from build123d import *

# Parameters (mm, degrees)
SKETCH1_W           = 29.9
SKETCH1_H           = 12.55
SKETCH1_R           = 1.5
BOSS_EXTRUDE1_DEPTH = 3.175
SKETCH2_W           = 29.9
SKETCH2_H           = 12.55
BOSS_EXTRUDE2_DEPTH = 3.175
BOSS_EXTRUDE3_DEPTH = 55.88
BOSS_EXTRUDE4_DEPTH = 3.175
SKETCH6_W           = 25.9
SKETCH6_H           = 8.55
CUT_EXTRUDE1_DEPTH  = 57.23
SKETCH7_W           = 23.9
SKETCH7_H           = 49.88
CUT_EXTRUDE2_DEPTH  = 23.211


with BuildPart() as part:
    # Sketch1 → Boss-Extrude1 (new body)
    # profile 1 of 3: a face of its own
    with BuildSketch(Plane.XY):
        with Locations((14.95, 6.275)):
            Rectangle(SKETCH1_W, SKETCH1_H)
    # profile 2 of 3: a face of its own
    with BuildSketch(Plane.XY):
        with BuildLine():
            Line((-5, 6.275), (0, 6.275))
            Line((0, 6.275), (0, 12.55))
            Line((0, 12.55), (-5, 12.55))
            ThreePointArc((-5, 12.55), (-8.1375, 9.4125), (-5, 6.275))
        make_face()
        with Locations((-5, 9.4125)):
            Circle(SKETCH1_R, mode=Mode.SUBTRACT)
    # profile 3 of 3: a face of its own
    with BuildSketch(Plane.XY):
        with BuildLine():
            Line((29.9, 12.55), (29.9, 6.275))
            Line((29.9, 6.275), (34.9, 6.275))
            ThreePointArc((34.9, 6.275), (38.0375, 9.4125), (34.9, 12.55))
            Line((34.9, 12.55), (29.9, 12.55))
        make_face()
        with Locations((34.9, 9.4125)):
            Circle(SKETCH1_R, mode=Mode.SUBTRACT)
    extrude(amount=BOSS_EXTRUDE1_DEPTH)

    # Sketch2 → Boss-Extrude2 (add)
    with BuildSketch(Plane.XY.offset(3.175)):
        with Locations((14.95, 6.275)):
            Rectangle(SKETCH2_W, SKETCH2_H)
    extrude(amount=BOSS_EXTRUDE2_DEPTH)

    # Sketch3 → Boss-Extrude3 (add)
    with BuildSketch(Plane(origin=(0, 0, 0), x_dir=(-1, 0, 0), z_dir=(0, 0, -1))):
        Polygon((-29.9, 0), (-29.9, -15.661), (0, -15.661), (0, 12.55), (-29.9, 12.55), align=None)
    extrude(amount=BOSS_EXTRUDE3_DEPTH)

    # Sketch5 → Boss-Extrude4 (add)
    with BuildSketch(Plane.XY.offset(3.175)):
        with BuildLine():
            Line((32.9, 6.275), (29.9, 6.275))
            Line((29.9, 6.275), (29.9, 3.275))
            ThreePointArc((29.9, 3.275), (30.778679656, 5.396320344), (32.9, 6.275))
        make_face()
        with BuildLine():
            Line((0, 6.275), (-3, 6.275))
            ThreePointArc((-3, 6.275), (-0.878679656, 5.396320344), (0, 3.275))
            Line((0, 3.275), (0, 6.275))
        make_face()
    extrude(amount=-BOSS_EXTRUDE4_DEPTH)

    # Sketch6 → Cut-Extrude1 (cut)
    with BuildSketch(Plane.XY.offset(6.35)):
        with Locations((14.95, 6.275)):
            Rectangle(SKETCH6_W, SKETCH6_H)
    extrude(amount=-CUT_EXTRUDE1_DEPTH, mode=Mode.SUBTRACT)

    # Sketch7 → Cut-Extrude2 (cut)
    with BuildSketch(Plane(origin=(0, 12.55, 0), x_dir=(1, 0, 0), z_dir=(0, 1, 0))):
        with Locations((14.95, 27.94)):
            Rectangle(SKETCH7_W, SKETCH7_H)
    extrude(amount=-CUT_EXTRUDE2_DEPTH, mode=Mode.SUBTRACT)


solid = part.part
Work out the finished part from the listing and answer in its coordinate system (mm). A direction names the side the tool comes from. Coordinates: 2 decimals unless noted, no trailing zeros. Order: outer loops, then holes, each group sorted by start corner. A loop starts at its lowest first (then second) coordinate and runs counter-clockwise, first axis right, second up. Notation, with made-up numbers: (79.5, 27) - (103.5, 27) arc R34 ccw to (103.5, 65) - close; hole circle Ø1 at (34.25, 0). An arc over 180 degrees is marked (long way). Put each result on its own line as item: value. Start each with the question number.
1) Find section C-C (z = -8.5). Give the vertices of the cut face in (x, y), plus the area to 3 significant figures.
2) Find section A-A (x = 21.5). Give the vertices of the cut face in (y, z), plus the area to 3 significant figures.
3) Find section B-B (y = -3.25). Give the vertices of the cut face in (x, z), plus the area to 3 significant figures.
4) For faces 1 (the flat face through (15, 10.55, -1)), 2 (the flat face through (-4, 6.275, 2)), 3 (the flat face through (15, 0, 3)), determine the directions among +Z, -Z, +X, -X, +Y, -Y from which every point of the face is accessible in a straight line to the end or side of a thin tool.
5) Find the intervals of material crossed by line 1 (X direction, y = 8.75, z = -40); line 2 (X direction, y = -4.25, z = -5); line 3 (Z direction, x = 16, y = 11), in increasing order. Write a range as from..to.
6) Flat-ended cylindrical pins translate along their axes: pin 1 (2 mm diameter, centred on y = -7.5, z = -20.5, fed in from -X); pin 2 (2.5 mm diameter, centred on x = 35.5, y = 7.5, fed in from +Z) (3 decimals); pin 3 (3 mm diameter, centred on x = 13.5, z = 2, fed in from -Y); pin 4 (2.5 mm diameter, centred on x = -5, y = 9.41, fed in from -Z). Find the tip coordinate at first contact, or state that the pin passes through.
7) For a pull along X with two mould halves and no side action, classify faces 4 (the flat face through (15, -4, -3)), 5 (the cylindrical face through (-5.2, 10.9, 1.6)), 6 (the flat face through (0, -2, -24)), 7 (the flat face through (2, 12.55, -15)) as released by +X, released by -X, zero draft, split by the parting line, or undercut.
Results list:
1. outline: (0, -15.66) - (29.9, -15.66) - (29.9, 12.55) - (26.9, 12.55) - (26.9, 10.55) - (27.9, 10.55) - (27.9, 2) - (26.9, 2) - (26.9, -10.66) - (3, -10.66) - (3, 2) - (2, 2) - (2, 10.55) - (3, 10.55) - (3, 12.55) - (0, 12.55) - close
1. area: 272 mm^2
2. outline: (-15.66, -55.88) - (12.55, -55.88) - (12.55, -52.88) - (-10.66, -52.88) - (-10.66, -3) - (2, -3) - (2, 6.35) - (0, 6.35) - (0, 0) - (-15.66, 0) - close; (10.55, -3) - (12.55, -3) - (12.55, 6.35) - (10.55, 6.35) - close
2. area: 418 mm^2
3. outline: (0, -55.88) - (29.9, -55.88) - (29.9, 0) - (0, 0) - close; hole (3, -52.88) - (26.9, -52.88) - (26.9, -3) - (3, -3) - close
3. area: 479 mm^2
4. face 1: +Z
4. face 2: +Z, -Z, -X, -Y
4. face 3: +Z, +X, -X, -Y
5. line 1: x = 0..2, 27.9..29.9
5. line 2: x = 0..3, 26.9..29.9
5. line 3: z = -55.88..-52.88, -3..6.35
6. pin 1: stops at x = 0
6. pin 2: stops at z = 3.175
6. pin 3: stops at y = 0
6. pin 4: passes through
7. face 4: undercut
7. face 5: undercut
7. face 6: released by -X
7. face 7: zero draft
